Build history of the part. All positions in model axes, mm. Face numbers are marked on the shaded views. A direction names the side the tool comes from. Give positions to 0.01 mm unless a question says otherwise; leave off trailing zeros. Loops run counter-clockwise (first coordinate to the right, second up) from the corner with the lowest first, then second, coordinate; pieces in that order, holes last. Notation, with made-up numbers: (81, 78.25) -> (113, 78.25) arc R18 ccw to (113, 89.25) -> close; hole circle Ø2 at (11, 31). An arc over 180 degrees is marked (long way). One line per question, with ' | ' between items. Start each with the question number.
(1) Mould opens along Z. For the marked faces 1, 2 and 3 say: pulls with the +Z half, pulls with the -Z half, needs draft (parallel to the pull), parting line crosses it, or undercut.
(2) Drill centre lines: L1, parallel to Z at x = -25, y = 2; L2, parallel to X at y = 1, z = 1.25; L3, parallel to Y at x = 16.5, z = 5.25. Where is each one in solid material? Low to high. Write a range as from..to.
(3) Flat gauge pins, fed straight in: pin 1 Ø2.5 at (y, z) = (6.5, 12.5) entering from -X; pin 2 Ø0.9 at (x, z) = (-24.5, 3) entering from -Y; pin 3 Ø6.5 at (x, y) = (-25, 5.5) entering from +Z; pin 4 Ø3.5 at (x, z) = (-21.5, 13) entering from +Y. Where does each tip first touch, or does it go through?
(4) Slice it at B-B, the plane y = 4.25. Write the cut outline in (x, z).
(5) 3-axis set-ups, long thin cutter, end or side, ignore diameter. For the marked faces 4, 5 and 6: which of +Z, -Z, +X, -X, +Y, -Y reach the whole face in a straight line?
(6) Slice it at C-C, the plane z = 20. Write the cut outline in (x, y).
(7) Slice it at D-D, the plane x = 11. Write the cut outline in (y, z), then the cut area to 3 significant figures.
(8) Slice it at A-A, the plane x = -21. Write the cut outline in (y, z), then the cut area to 3 significant figures.
Autodesk Inventor part; units mm, degrees
ref_plane "YZ Plane" through (0, 0, 0) normal (1, 0, 0) x (0, 1, 0)
ref_plane "XZ Plane" through (0, 0, 0) normal (0, 1, 0) x (-1, 0, 0)
ref_plane "XY Plane" through (0, 0, 0) normal (0, 0, 1) x (1, 0, 0)
sketch "スケッチ1" plane through (0, 0, 0) normal (0, 0, 1) x (1, 0, 0)
  line L0 (-19.5, 11) -> (-19.5, 0)
  line L1 (-19.5, 0) -> (19.5, 0)
  line L2 (19.5, 0) -> (19.5, 8)
  line L3 (19.5, 8) -> (-2.5, 8)
  line L4 (-2.5, 8) -> (-7.5, 11)
  line L5 (-7.5, 11) -> (-19.5, 11)
  point P0 (0, 0)
  point P1 (0, 0)
  dimension "d0" = 8
  dimension "d1" = 11
  dimension "d2" = 39
  dimension "d3" = 12
  dimension "d4" = 22
extrude "押し出し1" add sketch "スケッチ1" along normal blind 22
fillet "フィレット1" radius 1 16 edges at (0, 0, 22) (8.5, 8, 22) (19.5, 4, 22) (-19.5, 0, 11) (0, 0, 0) (19.5, 0, 11) (19.5, 4, 0) (19.5, 8, 11) (-5, 9.5, 22) (8.5, 8, 0) (-5, 9.5, 0) (-13.5, 11, 22) (-19.5, 5.5, 22) (-13.5, 11, 0) (-19.5, 5.5, 0) (-19.5, 11, 11)
fillet "フィレット1" radius 4 2 edges at (-7.5, 11, 11) (-2.5, 8, 11)
sketch "スケッチ2" plane through (-19.5, 1, 1) normal (-1, 0, 0) x (0, 0, 1)
  line L0 (0, 0) -> (0, 9)
  line L1 (20, 0) -> (0, 0)
  line L2 (20, 9) -> (20, 0)
  line L3 (0.5347, 8.5347) -> (0.5347, 0.5347)
  line L4 (0.5347, 0.5347) -> (19.4653, 0.5347)
  line L5 (19.4653, 0.5347) -> (19.4653, 8.5)
  line L6 (0.5347, 8.5347) -> (3.5347, 8.5347)
  line L7 (3.5347, 8.5347) -> (3.5347, 0.5347)
  line L8 (3.5347, 0.5347) -> (0.5347, 0.5347)
  line L9 (0.5347, 0.5347) -> (0.5347, 8.5347)
  line L10 (3.7208, 8.5347) -> (6.7208, 8.5347)
  line L11 (6.7208, 8.5347) -> (6.7208, 0.5347)
  line L12 (6.7208, 0.5347) -> (3.7208, 0.5347)
  line L13 (3.7208, 0.5347) -> (3.7208, 8.5347)
  line L14 (6.9069, 8.5347) -> (9.9069, 8.5347)
  line L15 (9.9069, 8.5347) -> (9.9069, 0.5347)
  line L16 (9.9069, 0.5347) -> (6.9069, 0.5347)
  line L17 (6.9069, 0.5347) -> (6.9069, 8.5347)
  line L18 (10.0931, 8.5347) -> (13.0931, 8.5347)
  line L19 (13.0931, 8.5347) -> (13.0931, 0.5347)
  line L20 (13.0931, 0.5347) -> (10.0931, 0.5347)
  line L21 (10.0931, 0.5347) -> (10.0931, 8.5347)
  line L22 (13.2792, 8.5347) -> (16.2792, 8.5347)
  line L23 (16.2792, 8.5347) -> (16.2792, 0.5347)
  line L24 (16.2792, 0.5347) -> (13.2792, 0.5347)
  line L25 (13.2792, 0.5347) -> (13.2792, 8.5347)
  line L26 (16.4653, 8.5347) -> (19.4653, 8.5347)
  line L27 (19.4653, 8.5347) -> (19.4653, 0.5347)
  line L28 (19.4653, 0.5347) -> (16.4653, 0.5347)
  line L29 (16.4653, 0.5347) -> (16.4653, 8.5347)
  line L30 (3.5347, 8.5347) -> (3.7208, 8.5347)
  line L31 (6.7208, 8.5347) -> (6.9069, 8.5347)
  line L32 (9.9069, 8.5347) -> (10.0931, 8.5347)
  line L33 (13.0931, 8.5347) -> (13.2792, 8.5347)
  line L34 (16.2792, 8.5347) -> (16.4653, 8.5347)
  point P0 (-1, -1)
  dimension "d9" = 8
  dimension "d11" = 0.5347
  dimension "d12" = 3
extrude "押し出し2" add sketch "スケッチ2" along normal blind 8 contours L6 L7 L4 L3 | L10 L11 L4 L13 | L14 L15 L4 L17 | L18 L19 L4 L21 | L22 L23 L4 L25 | L26 L27 L5 L4 L29
sketch "スケッチ4" plane through (-27.5, 1, 1) normal (-1, 0, 0) x (0, 0, 1)
  line L0 (0.5347, 8.5347) -> (0.5347, 0.5347)
  line L1 (6.7208, 0.5347) -> (6.7208, 8.5347)
  line L2 (6.7208, 8.5347) -> (3.7208, 8.5347)
  line L3 (3.7208, 8.5347) -> (3.7208, 0.5347)
  line L4 (3.7208, 0.5347) -> (6.7208, 0.5347)
  line L5 (9.9069, 0.5347) -> (9.9069, 8.5347)
  line L6 (9.9069, 8.5347) -> (6.9069, 8.5347)
  line L7 (6.9069, 8.5347) -> (6.9069, 0.5347)
  line L8 (6.9069, 0.5347) -> (9.9069, 0.5347)
  line L9 (13.0931, 0.5347) -> (13.0931, 8.5347)
  line L10 (13.0931, 8.5347) -> (10.0931, 8.5347)
  line L11 (10.0931, 8.5347) -> (10.0931, 0.5347)
  line L12 (10.0931, 0.5347) -> (13.0931, 0.5347)
  line L13 (16.2792, 0.5347) -> (16.2792, 8.5347)
  line L14 (16.2792, 8.5347) -> (13.2792, 8.5347)
  line L15 (13.2792, 8.5347) -> (13.2792, 0.5347)
  line L16 (13.2792, 0.5347) -> (16.2792, 0.5347)
  line L17 (19.4653, 0.5347) -> (19.4653, 8.5347)
  line L18 (19.4653, 8.5347) -> (16.4653, 8.5347)
  line L19 (16.4653, 8.5347) -> (16.4653, 0.5347)
  line L20 (16.4653, 0.5347) -> (19.4653, 0.5347)
  line L21 (1.0347, 3.5347) -> (1.0347, 5.5347)
  line L22 (1.0347, 1.0347) -> (1.0347, 3.0347)
  line L23 (1.0347, 7.3573) -> (0.5347, 7.3573)
  line L24 (1.3567, 6.0347) -> (1.3567, 5.5347)
  line L25 (1.3567, 3.5347) -> (1.3567, 3.0347)
  circle A0 centre (2.0347, 2.0347) radius 0.75
  circle A1 centre (2.0347, 4.5347) radius 0.75
  circle A2 centre (2.0347, 7.0347) radius 0.75
  circle A3 centre (5.2208, 7.0347) radius 0.75
  circle A4 centre (5.2208, 4.5347) radius 0.75
  circle A5 centre (5.2208, 2.0347) radius 0.75
  circle A6 centre (8.4069, 7.0347) radius 0.75
  circle A7 centre (8.4069, 4.5347) radius 0.75
  circle A8 centre (8.4069, 2.0347) radius 0.75
  circle A9 centre (11.5931, 2.0347) radius 0.75
  circle A10 centre (11.5931, 4.5347) radius 0.75
  circle A11 centre (11.5931, 7.0347) radius 0.75
  circle A12 centre (14.7792, 7.0347) radius 0.75
  circle A13 centre (14.7792, 4.5347) radius 0.75
  circle A14 centre (14.7792, 2.0347) radius 0.75
  circle A15 centre (17.9653, 2.0347) radius 0.75
  circle A16 centre (17.9653, 4.5347) radius 0.75
  circle A17 centre (17.9653, 7.0347) radius 0.75
  point P0 (-1, -1)
  dimension "d17" = 1.5
extrude "押し出し3" add sketch "スケッチ4" along normal blind 4 contours A0 | A1 | A2 | A3 | A4 | A5 | A6 | A7 | A8 | A9 | A10 | A11 | A12 | A13 | A14 | A15 | A16 | A17
sketch "スケッチ5" plane through (-31.5, 3.0347, 6.2208) normal (-1, 0, 0) x (0, 0, 1)
  line L0 (14.2445, 6.5) -> (14.2445, -1.5)
  circle A0 centre (12.7445, 2.5) radius 0.75
  circle A1 centre (12.7445, 0) radius 0.75
  circle A2 centre (12.7445, 5) radius 0.75
  line L1 (14.2445, -1.5) -> (14.2445, 6.5)
  line L2 (14.2445, 6.5) -> (11.2445, 6.5)
  line L3 (11.2445, 6.5) -> (11.2445, -1.5)
  line L4 (11.2445, -1.5) -> (14.2445, -1.5)
  circle A3 centre (0, 2.5) radius 0.75
  circle A4 centre (0, 5) radius 0.75
  circle A5 centre (0, 0) radius 0.75
  line L5 (1.5, -1.5) -> (1.5, 6.5)
  line L6 (1.5, 6.5) -> (-1.5, 6.5)
  line L7 (-1.5, 6.5) -> (-1.5, -1.5)
  line L8 (-1.5, -1.5) -> (1.5, -1.5)
  point P0 (-6.2208, -3.0347)
extrude "押し出し4" cut sketch "スケッチ5" against normal blind 12 contours L0 L4 L3 L2 | A0 | A1 | A2 | A3 | A4 | A5 | L8 L7 L6 L5
properties part number "受信機"
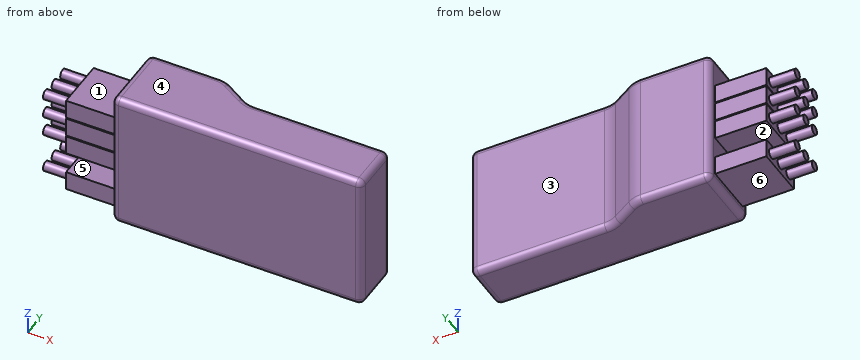
Final values:
1) face 1: pulls with the +Z half | face 2: undercut | face 3: needs draft
2) L1: 1.53..4.53, 7.91..10.91, 11.09..14.09, 14.28..17.28 | L2: -19.5..19.5 | L3: 0..8
3) pin 1: x = -31.5 | pin 2: y = 1.53 | pin 3: z = 17.28 | pin 4: y = 9.53
4) outline: (-27.5, 1.53) -> (-19.5, 1.53) -> (-19.5, 1) arc R1 ccw to (-18.5, 0) -> (18.5, 0) arc R1 ccw to (19.5, 1) -> (19.5, 21) arc R1 ccw to (18.5, 22) -> (-18.5, 22) arc R1 ccw to (-19.5, 21) -> (-19.5, 17.28) -> (-27.5, 17.28) -> (-27.5, 14.28) -> (-19.5, 14.28) -> (-19.5, 14.09) -> (-27.5, 14.09) -> (-27.5, 11.09) -> (-19.5, 11.09) -> (-19.5, 10.91) -> (-27.5, 10.91) -> (-27.5, 7.91) -> (-19.5, 7.91) -> (-19.5, 4.53) -> (-27.5, 4.53) -> close
5) face 4: +Z, +X, -X, +Y, -Y | face 5: -X, +Y, -Y | face 6: -Z, -X, +Y, -Y
6) outline: (-19.5, 1) arc R1 ccw to (-18.5, 0) -> (18.5, 0) arc R1 ccw to (19.5, 1) -> (19.5, 7) arc R1 ccw to (18.5, 8) -> (-1.39, 8) arc R4 cw to (-3.45, 8.57) -> (-6.55, 10.43) arc R4 ccw to (-8.61, 11) -> (-18.5, 11) arc R1 ccw to (-19.5, 10) -> close
7) outline: (0, 1) arc R1 ccw to (1, 0) -> (7, 0) arc R1 ccw to (8, 1) -> (8, 21) arc R1 ccw to (7, 22) -> (1, 22) arc R1 ccw to (0, 21) -> close | area: 175 mm2
8) outline: (1.53, 1.53) -> (9.53, 1.53) -> (9.53, 4.53) -> (1.53, 4.53) -> close; (1.53, 7.91) -> (9.53, 7.91) -> (9.53, 10.91) -> (1.53, 10.91) -> close; (1.53, 11.09) -> (9.53, 11.09) -> (9.53, 14.09) -> (1.53, 14.09) -> close; (1.53, 14.28) -> (9.53, 14.28) -> (9.53, 17.28) -> (1.53, 17.28) -> close | area: 96.0 mm2
